Input: part model. Units: mm. Frame: model coordinates. A direction names the side the tool comes from. Coordinates: 2 decimals unless noted, no trailing zeros. Order: outer loops, then holes, each group sorted by start corner. A loop starts at its lowest first (then second) coordinate and runs counter-clockwise, first axis right, second up.
from build123d import *

# Parameters (mm, degrees)
F0_R     = 6
F0_R_2   = 3.25
F1_DEPTH = 1.5
F2_R     = 6
F2_R_2   = 4.3
F3_DEPTH = 2
F4_W     = 5
F4_H     = 3.923344
F5_DEPTH = 3
F6_SIZE  = 0.5


with BuildPart() as f1:
    # F0 (on Top) → F1 (new body)
    with BuildSketch(Plane.XY):
        Circle(F0_R)
        Circle(F0_R_2, mode=Mode.SUBTRACT)
    extrude(amount=F1_DEPTH)

    # F2 (on face) → F3 (join)
    with BuildSketch(Plane.XY.offset(1.5)):
        Circle(F2_R)
        Circle(F2_R_2, mode=Mode.SUBTRACT)
    extrude(amount=F3_DEPTH)

    # F4 (on face) → F5 (cut)
    with BuildSketch(Plane.XY.offset(3.5)):
        with Locations((0, 4.038328)):
            Rectangle(F4_W, F4_H)
    extrude(amount=-F5_DEPTH, mode=Mode.SUBTRACT)

    # F6
    f6_edges = [f1.edges().sort_by_distance(p)[0] for p in [
        (0, -4.3, 3.5),
    ]]
    chamfer(f6_edges, length=F6_SIZE)


solid = f1.part
Item 1: Ray query, probe 1 along X at (y, z) = (0, 1.05); probe 2 along Z at (x, y) = (1.25, 3.5). Return the intervals inside material, ascending.
Response values:
probe 1: x = -6 to -3.25, 3.25 to 6
probe 2: z = 0 to 0.5
Item 2: Pin query (flat end, axial travel): pin 1 Ø2 at (x, y) = (-1, 4) entering from +Z. Return the tip coordinate at first contact, or that it passes through.
Response values:
pin 1: stops at z = 0.5
Item 3: Cut plane C-C on z = 0.2. Return loops of the section in (x, y).
Response values:
outline: circle Ø12 at (0, 0); hole circle Ø6.5 at (0, 0)
Item 4: Cut plane D-D on z = 1.1. Return loops of the section in (x, y).
Response values:
outline: (-2.5, 2.08) - (-2.5, 5.45) arc R6 ccw (long way) to (2.5, 5.45) - (2.5, 2.08) arc R3.25 cw (long way) to start
Item 5: Cut plane B-B on x = 0. Return loops of the section in (y, z).
Response values:
outline: (-6, 0) - (-3.25, 0) - (-3.25, 1.5) - (-4.3, 1.5) - (-4.3, 3) - (-4.8, 3.5) - (-6, 3.5) - close; (3.25, 0) - (6, 0) - (6, 0.5) - (3.25, 0.5) - close
Item 6: Cut plane A-A on y = 0. Return loops of the section in (x, z), then the cut area to 3 significant figures.
Response values:
outline: (-6, 0) - (-3.25, 0) - (-3.25, 1.5) - (-4.3, 1.5) - (-4.3, 3) - (-4.8, 3.5) - (-6, 3.5) - close; (3.25, 0) - (6, 0) - (6, 3.5) - (4.8, 3.5) - (4.3, 3) - (4.3, 1.5) - (3.25, 1.5) - close
area: 14.8 mm2
Item 7: Access query for faces 1 (the face through (0, -5, 3.5)), 2 (the face through (2.5, 4, 2)), 3 (the face through (0, -4, 1.5)). Directions: +Z, -Z, +X, -X, +Y, -Y. A direction counts if a zero-diameter tool reaches every point of the face in a straight line with its end or side. Return the directions, or none.
Response values:
face 1: +Z, +X, -X, +Y, -Y
face 2: +Z, +Y
face 3: +Z
Item 8: Draft query along Y for faces 4 (the face through (-1.301, -5.857, 1.726)), 5 (the face through (-0.705, -3.173, 0.74)), 6 (the face through (-2.5, 4, 2)). Return one class per face: pulls with the +Y half, pulls with the -Y half, needs draft (parallel to the pull), parting line crosses it, or undercut.
Response values:
face 4: parting line crosses it
face 5: undercut
face 6: needs draft
